Could you check a few things on this model? Use its own coordinates, in mm. A direction names the side the tool comes from. Round coordinates to 2 decimals unless told otherwise and drop trailing zeros. Loops run counter-clockwise (first coordinate to the right, second up) from the corner with the lowest first, then second, coordinate; pieces in that order, holes last. Notation, with made-up numbers: (-27.75, 34.5) - (-1.75, 34.5) arc R9 ccw to (-1.75, 44.5) - close; hole circle Ø11 at (75.5, 79.25). An arc over 180 degrees is marked (long way). Put each result on its own line as item: value. Start each with the question number.
from build123d import *

# Parameters (mm, degrees)
SKETCH1_R               = 5
BOSS_EXTRUDE1_DEPTH     = 20
SKETCH2_R               = 4.25
CUT_EXTRUDE1_DEPTH      = 17.5
SKETCH3_R               = 1.25
CUT_EXTRUDE2_DEPTH      = 2.5
CUT_EXTRUDE3_DEPTH      = 10
CUT_EXTRUDE3_DEPTH_BACK = 10
SKETCH4_R               = 1.1


with BuildPart() as part:
    # Sketch1 → Boss-Extrude1 (new body)
    with BuildSketch(Plane(origin=(0, 0, 0), x_dir=(1, 0, 0), z_dir=(0, 1, 0))):
        with Locations(Location((0, 0, 0), (0, 0, 270))):
            Circle(SKETCH1_R)
    extrude(amount=BOSS_EXTRUDE1_DEPTH)

    # Sketch2 → Cut-Extrude1 (cut)
    with BuildSketch(Plane(origin=(0, 20, 0), x_dir=(1, 0, 0), z_dir=(0, 1, 0))):
        with Locations(Location((0, 0, 0), (0, 0, 270))):
            Circle(SKETCH2_R)
    extrude(amount=-CUT_EXTRUDE1_DEPTH, mode=Mode.SUBTRACT)

    # Sketch3 → Cut-Extrude2 (cut)
    with BuildSketch(Plane.XZ):
        with Locations(Location((0, 0, 0), (0, 0, 270))):
            Circle(SKETCH3_R)
    extrude(amount=-CUT_EXTRUDE2_DEPTH, mode=Mode.SUBTRACT)

    # Sketch4 → Cut-Extrude3 (cut, two sides: drawn at the far end of the back side and taken through both)
    with BuildSketch(Plane.XY.offset(-CUT_EXTRUDE3_DEPTH_BACK)):
        with Locations(Location((0, 12.5, 0), (0, 0, 180))):
            Circle(SKETCH4_R)
    extrude(amount=CUT_EXTRUDE3_DEPTH + CUT_EXTRUDE3_DEPTH_BACK, mode=Mode.SUBTRACT)


solid = part.part
Item 1: Suppose I cut it at D-D, the plane y = 5.75. List the corners of the cut face in (x, z) for me, then the cut area to 3 significant figures.
Item 2: Thinking about a two-plate mould opening in X: for faces 1 (the face through (1.5, 9.86, 4.77)), 2 (the face through (1.277, 11.372, 4.054)), 3 (the face through (-1, 0, 1)), 4 (the face through (-1.22, 1.23, 0.27)), which applies, released by +X, released by -X, zero draft, split by the parting line, or undercut?
Item 3: Suppose I cut it at C-C, the plane y = 12.5. List the corners of the cut face in (x, z) for me, then the cut area to 3 significant figures.
Item 4: I need wall thicknesses on line 1 (X direction, y = 1.3, z = 0); line 2 (Y direction, x = 0, z = 4.35); line 3 (X direction, y = 11.75, z = 0). Which ranges of each line are inside material? Lowest first, please. Write a range as from..to.
Item 5: Suppose I cut it at B-B, the plane z = 0. List the corners of the cut face in (x, y) for me, then the cut area to 3 significant figures.
Item 6: On a 3-axis mill with a long thin cutter (end or side, diameter ignored), from which of +Z, -Z, +X, -X, +Y, -Y can I reach the whole of each face in a straight line? I mean faces 5 (the face through (-1, 2.5, 1)), 6 (the face through (-4, 20, -2)). Say none if no direction works.
Item 7: Suppose I cut it at A-A, the plane x = 0. List the corners of the cut face in (y, z) for me.
Item 8: Will these pins go through, and if not, where does the flat tip stop? P1, Ø2.5, axis at x = 2, z = 1.5, coming from the +Y side; P2, Ø1.5, axis at y = 6, z = 3.5, coming from the +X side; P3, Ø2, axis at x = 0, z = 0, coming from the +Y side; P4, Ø5, axis at y = 16.5, z = -3.5, coming from the +X side.
Numbers:
1. outline: circle Ø10 at (0, 0); hole circle Ø8.5 at (0, 0)
1. area: 21.8 mm^2
2. face 1: split by the parting line
2. face 2: undercut
2. face 3: zero draft
2. face 4: undercut
3. outline: (-1.1, -4.88) - (-1.1, -4.11) arc R4.25 cw to (-1.1, 4.11) - (-1.1, 4.88) arc R5 ccw to start; (1.1, -4.88) arc R5 ccw to (1.1, 4.88) - (1.1, 4.11) arc R4.25 cw to (1.1, -4.11) - close
3. area: 18.5 mm^2
4. line 1: -5..-1.25, 1.25..5
4. line 2: 0..11.4, 13.6..20
4. line 3: -5..-4.25, 4.25..5
5. outline: (-5, 0) - (-1.25, 0) - (-1.25, 2.5) - (-4.25, 2.5) - (-4.25, 20) - (-5, 20) - close; (1.25, 0) - (5, 0) - (5, 20) - (4.25, 20) - (4.25, 2.5) - (1.25, 2.5) - close
5. area: 45.0 mm^2
6. face 5: +Y
6. face 6: +Z, -Z, +X, -X, +Y
7. outline: (0, -5) - (11.4, -5) - (11.4, -4.25) - (2.5, -4.25) - (2.5, -1.25) - (0, -1.25) - close; (0, 1.25) - (2.5, 1.25) - (2.5, 4.25) - (11.4, 4.25) - (11.4, 5) - (0, 5) - close; (13.6, -5) - (20, -5) - (20, -4.25) - (13.6, -4.25) - close; (13.6, 4.25) - (20, 4.25) - (20, 5) - (13.6, 5) - close
8. P1: y = 2.5
8. P2: x = 4.18
8. P3: through
8. P4: x = 4.9
